```python
from build123d import *

# Parameters (mm, degrees)
SKETCH_1_W          = 70
SKETCH_1_H          = 60
EXTRUDE_1_DEPTH     = 5
SKETCH_2_W          = 38
SKETCH_2_H          = 38
EXTRUDE_2_DEPTH     = 5
CUT_EXTRUDE_1_REACH = 49.17
SKETCH_3_R          = 1.1
SKETCH_4_R          = 3
CUT_EXTRUDE_2_DEPTH = 8.5
CUT_EXTRUDE_3_REACH = 48.368
SKETCH_5_R          = 1.5
SKETCH_6_R          = 3
CUT_EXTRUDE_4_DEPTH = 3.5
CUT_EXTRUDE_5_DEPTH = 41.5


with BuildPart() as part:
    # 草图1 → 凸台-拉伸1 (new body)
    with BuildSketch(Plane(origin=(0, 0, 0), x_dir=(1, 0, 0), z_dir=(0, 1, 0))):
        Rectangle(SKETCH_1_W, SKETCH_1_H)
    extrude(amount=EXTRUDE_1_DEPTH)

    # 草图2 → 凸台-拉伸2 (add)
    with BuildSketch(Plane(origin=(0, 5, 0), x_dir=(1, 0, 0), z_dir=(0, 1, 0))):
        with Locations((-5, 0)):
            Rectangle(SKETCH_2_W, SKETCH_2_H)
    extrude(amount=EXTRUDE_2_DEPTH)

    # 草图3 → 切除-拉伸1 (cut, up to next)
    with BuildSketch(Plane(origin=(0, 10, 0), x_dir=(1, 0, 0), z_dir=(0, 1, 0)), mode=Mode.PRIVATE) as cut_extrude_1_sk1:
        with Locations(Location((-19, 14, 0), (0, 0, 270))):
            Circle(SKETCH_3_R)
    cut_extrude_1_tool1 = extrude(cut_extrude_1_sk1.sketch, amount=-CUT_EXTRUDE_1_REACH, mode=Mode.PRIVATE) & part.part
    # 草图3 → 切除-拉伸1 (cut, up to next)
    with BuildSketch(Plane(origin=(0, 10, 0), x_dir=(1, 0, 0), z_dir=(0, 1, 0)), mode=Mode.PRIVATE) as cut_extrude_1_sk2:
        with Locations(Location((9, 14, 0), (0, 0, 270))):
            Circle(SKETCH_3_R)
    cut_extrude_1_tool2 = extrude(cut_extrude_1_sk2.sketch, amount=-CUT_EXTRUDE_1_REACH, mode=Mode.PRIVATE) & part.part
    # 草图3 → 切除-拉伸1 (cut, up to next)
    with BuildSketch(Plane(origin=(0, 10, 0), x_dir=(1, 0, 0), z_dir=(0, 1, 0)), mode=Mode.PRIVATE) as cut_extrude_1_sk3:
        with Locations(Location((-19, -14, 0), (0, 0, 270))):
            Circle(SKETCH_3_R)
    cut_extrude_1_tool3 = extrude(cut_extrude_1_sk3.sketch, amount=-CUT_EXTRUDE_1_REACH, mode=Mode.PRIVATE) & part.part
    # 草图3 → 切除-拉伸1 (cut, up to next)
    with BuildSketch(Plane(origin=(0, 10, 0), x_dir=(1, 0, 0), z_dir=(0, 1, 0)), mode=Mode.PRIVATE) as cut_extrude_1_sk4:
        with Locations(Location((9, -14, 0), (0, 0, 270))):
            Circle(SKETCH_3_R)
    cut_extrude_1_tool4 = extrude(cut_extrude_1_sk4.sketch, amount=-CUT_EXTRUDE_1_REACH, mode=Mode.PRIVATE) & part.part
    add(cut_extrude_1_tool1.solids().sort_by_distance((-19, 10, -14))[0], mode=Mode.SUBTRACT)
    add(cut_extrude_1_tool2.solids().sort_by_distance((9, 10, -14))[0], mode=Mode.SUBTRACT)
    add(cut_extrude_1_tool3.solids().sort_by_distance((-19, 10, 14))[0], mode=Mode.SUBTRACT)
    add(cut_extrude_1_tool4.solids().sort_by_distance((9, 10, 14))[0], mode=Mode.SUBTRACT)

    # 草图4 → 切除-拉伸2 (cut)
    with BuildSketch(Plane.XZ):
        with Locations(Location((-19, -14, 0), (0, 0, 270))):
            Circle(SKETCH_4_R)
        with Locations(Location((-19, 14, 0), (0, 0, 270))):
            Circle(SKETCH_4_R)
        with Locations(Location((9, 14, 0), (0, 0, 270))):
            Circle(SKETCH_4_R)
        with Locations(Location((9, -14, 0), (0, 0, 270))):
            Circle(SKETCH_4_R)
    extrude(amount=-CUT_EXTRUDE_2_DEPTH, mode=Mode.SUBTRACT)

    # 草图5 → 切除-拉伸3 (cut, up to next)
    with BuildSketch(Plane(origin=(0, 5, 0), x_dir=(1, 0, 0), z_dir=(0, 1, 0)), mode=Mode.PRIVATE) as cut_extrude_3_sk1:
        with Locations(Location((-30, 25, 0), (0, 0, 270))):
            Circle(SKETCH_5_R)
    cut_extrude_3_tool1 = extrude(cut_extrude_3_sk1.sketch, amount=-CUT_EXTRUDE_3_REACH, mode=Mode.PRIVATE) & part.part
    # 草图5 → 切除-拉伸3 (cut, up to next)
    with BuildSketch(Plane(origin=(0, 5, 0), x_dir=(1, 0, 0), z_dir=(0, 1, 0)), mode=Mode.PRIVATE) as cut_extrude_3_sk2:
        with Locations(Location((30, 25, 0), (0, 0, 270))):
            Circle(SKETCH_5_R)
    cut_extrude_3_tool2 = extrude(cut_extrude_3_sk2.sketch, amount=-CUT_EXTRUDE_3_REACH, mode=Mode.PRIVATE) & part.part
    # 草图5 → 切除-拉伸3 (cut, up to next)
    with BuildSketch(Plane(origin=(0, 5, 0), x_dir=(1, 0, 0), z_dir=(0, 1, 0)), mode=Mode.PRIVATE) as cut_extrude_3_sk3:
        with Locations(Location((30, -25, 0), (0, 0, 270))):
            Circle(SKETCH_5_R)
    cut_extrude_3_tool3 = extrude(cut_extrude_3_sk3.sketch, amount=-CUT_EXTRUDE_3_REACH, mode=Mode.PRIVATE) & part.part
    # 草图5 → 切除-拉伸3 (cut, up to next)
    with BuildSketch(Plane(origin=(0, 5, 0), x_dir=(1, 0, 0), z_dir=(0, 1, 0)), mode=Mode.PRIVATE) as cut_extrude_3_sk4:
        with Locations(Location((-30, -25, 0), (0, 0, 270))):
            Circle(SKETCH_5_R)
    cut_extrude_3_tool4 = extrude(cut_extrude_3_sk4.sketch, amount=-CUT_EXTRUDE_3_REACH, mode=Mode.PRIVATE) & part.part
    add(cut_extrude_3_tool1.solids().sort_by_distance((-30, 5, -25))[0], mode=Mode.SUBTRACT)
    add(cut_extrude_3_tool2.solids().sort_by_distance((30, 5, -25))[0], mode=Mode.SUBTRACT)
    add(cut_extrude_3_tool3.solids().sort_by_distance((30, 5, 25))[0], mode=Mode.SUBTRACT)
    add(cut_extrude_3_tool4.solids().sort_by_distance((-30, 5, 25))[0], mode=Mode.SUBTRACT)

    # 草图6 → 切除-拉伸4 (cut)
    with BuildSketch(Plane.XZ):
        with Locations(Location((-30, -25, 0), (0, 0, 270))):
            Circle(SKETCH_6_R)
        with Locations(Location((30, -25, 0), (0, 0, 270))):
            Circle(SKETCH_6_R)
        with Locations(Location((30, 25, 0), (0, 0, 270))):
            Circle(SKETCH_6_R)
        with Locations(Location((-30, 25, 0), (0, 0, 270))):
            Circle(SKETCH_6_R)
    extrude(amount=-CUT_EXTRUDE_4_DEPTH, mode=Mode.SUBTRACT)

    # 草图7 → 切除-拉伸5 (cut)
    with BuildSketch(Plane(origin=(35, 0, 0), x_dir=(0, 0, -1), z_dir=(1, 0, 0))):
        with BuildLine():
            Line((2.55, 5), (2.55, 10))
            Line((2.55, 10), (-2.55, 10))
            Line((-2.55, 10), (-2.55, 5))
            ThreePointArc((-2.55, 5), (0, 2.45), (2.55, 5))
        make_face()
    extrude(amount=-CUT_EXTRUDE_5_DEPTH, mode=Mode.SUBTRACT)


solid = part.part
```
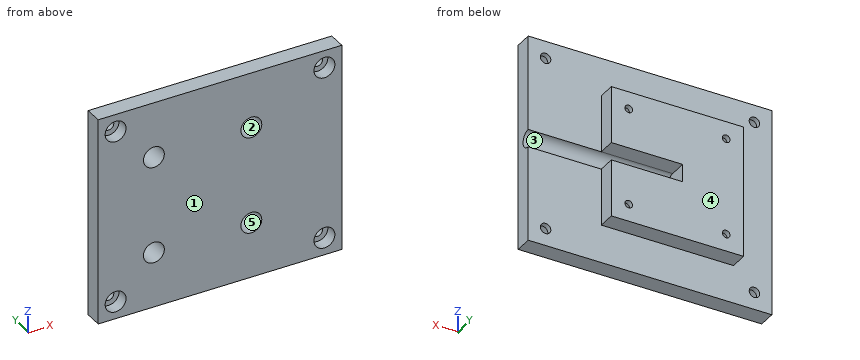
Geometry check sheet. Reference: the model listing, model coordinates, mm. Face numbers are marked on the shaded views. A direction names the side the tool comes from. Coordinates: 2 decimals unless noted, no trailing zeros. Loops run counter-clockwise (first coordinate to the right, second up) from the corner with the lowest first, then second, coordinate; pieces in that order, holes last. Notation, with made-up numbers: (-25.5, 30) - (-4.5, 30) arc R29 ccw to (-4.5, 59) - close; hole circle Ø3 at (-0.75, -25). An arc over 180 degrees is marked (long way). One line per item, written item: value. Start each with the question number.
(1) Mould release check, pull along X, two halves, no side actions. Record for the marked faces 4 and 5: released by +X, released by -X, zero draft, split by the parting line, or undercut.
(2) Tool access check on the marked faces 1, 2 and 3. Record the directions out of +Z, -Z, +X, -X, +Y, -Y that give a thin tool (end or side, any length) a straight path to the whole face; none if there is none.
(3) Depth check by flat-ended pin: P1, Ø1.8, axis at x = -19, z = 14, coming from the +Y side; P2, Ø1.8, axis at x = -19.5, z = -13, coming from the -Y side; P3, Ø1.5, axis at x = -12.5, y = 6.5, coming from the +Z side; P4, Ø5, axis at x = 30, z = -25, coming from the +Y side. Enter the tip coordinate at first touch or a pass-through.
(4) Cross-section at B-B on x = -30. Enter the section's corners in (y, z).
(5) Cross-section at C-C on z = -14. Enter the section's corners in (x, y).
(6) Material ranges on line 1 (X direction, y = 4.2, z = 25); line 2 (X direction, y = 9.6, z = 14); line 3 (Z direction, x = 6.5, y = 9.5), recorded low to high. Write a range as [from, to].
(7) Cross-section at D-D on x = -0.5. Enter the section's corners in (y, z).
(8) Cross-section at A-A on z = 25. Enter the section's corners in (x, y).
Results below:
1. face 4: zero draft
1. face 5: undercut
2. face 1: +Z, -Z, +X, -X, -Y
2. face 2: -Y
2. face 3: +X, +Y
3. P1: passes through
3. P2: stops at y = 8.5
3. P3: stops at z = 19
3. P4: stops at y = 5
4. outline: (0, -30) - (5, -30) - (5, -26.5) - (3.5, -26.5) - (3.5, -28) - (0, -28) - close; (0, -22) - (3.5, -22) - (3.5, -23.5) - (5, -23.5) - (5, 23.5) - (3.5, 23.5) - (3.5, 22) - (0, 22) - close; (0, 28) - (3.5, 28) - (3.5, 26.5) - (5, 26.5) - (5, 30) - (0, 30) - close
5. outline: (-35, 0) - (-22, 0) - (-22, 8.5) - (-20.1, 8.5) - (-20.1, 10) - (-24, 10) - (-24, 5) - (-35, 5) - close; (-17.9, 8.5) - (-16, 8.5) - (-16, 0) - (6, 0) - (6, 8.5) - (7.9, 8.5) - (7.9, 10) - (-17.9, 10) - close; (10.1, 8.5) - (12, 8.5) - (12, 0) - (35, 0) - (35, 5) - (14, 5) - (14, 10) - (10.1, 10) - close
6. line 1: x = [-35, -31.5], [-28.5, 28.5], [31.5, 35]
6. line 2: x = [-24, -20.1], [-17.9, 7.9], [10.1, 14]
6. line 3: z = [-19, -2.55], [2.55, 19]
7. outline: (0, -30) - (5, -30) - (5, -19) - (10, -19) - (10, -2.55) - (5, -2.55) arc R2.55 cw to (5, 2.55) - (10, 2.55) - (10, 19) - (5, 19) - (5, 30) - (0, 30) - close
8. outline: (-35, 0) - (-33, 0) - (-33, 3.5) - (-31.5, 3.5) - (-31.5, 5) - (-35, 5) - close; (-28.5, 3.5) - (-27, 3.5) - (-27, 0) - (27, 0) - (27, 3.5) - (28.5, 3.5) - (28.5, 5) - (-28.5, 5) - close; (31.5, 3.5) - (33, 3.5) - (33, 0) - (35, 0) - (35, 5) - (31.5, 5) - close
